```python
from build123d import *

# Parameters (mm, degrees)
SKETCH1_W           = 117.4
SKETCH1_H           = 25.4
BOSS_EXTRUDE1_DEPTH = 1.5875
SKETCH2_W           = 117.4
SKETCH2_H           = 1.5875
BOSS_EXTRUDE2_DEPTH = 23.8125
SKETCH3_R           = 2.54
CUT_EXTRUDE1_DEPTH  = 1.5875
SKETCH4_R           = 2.54
CUT_EXTRUDE2_DEPTH  = 1.5875
FILLET1_R           = 12.7
FILLET2_R           = 3.175


with BuildPart() as part:
    # Sketch1 → Boss-Extrude1 (new body)
    with BuildSketch(Plane.XY):
        with Locations((58.7, 0)):
            Rectangle(SKETCH1_W, SKETCH1_H)
    extrude(amount=BOSS_EXTRUDE1_DEPTH)

    # Sketch2 → Boss-Extrude2 (add)
    with BuildSketch(Plane.XY.offset(1.5875)):
        with Locations((58.7, -11.90625)):
            Rectangle(SKETCH2_W, SKETCH2_H)
    extrude(amount=BOSS_EXTRUDE2_DEPTH)

    # Sketch3 → Cut-Extrude1 (cut)
    with BuildSketch(Plane(origin=(0, -11.1125, 0), x_dir=(1, 0, 0), z_dir=(0, 1, 0))):
        with Locations(Location((12.7, -6.64845, 0), (0, 0, 270))):
            Circle(SKETCH3_R)
        with Locations(Location((104.6990032, -6.64845, 0), (0, 0, 270))):
            Circle(SKETCH3_R)
    extrude(amount=-CUT_EXTRUDE1_DEPTH, mode=Mode.SUBTRACT)

    # Sketch4 → Cut-Extrude2 (cut)
    with BuildSketch(Plane.XY.offset(1.5875)):
        with Locations((18.975, 3.175)):
            Circle(SKETCH4_R)
        with Locations((98.35, 3.175)):
            Circle(SKETCH4_R)
    extrude(amount=-CUT_EXTRUDE2_DEPTH, mode=Mode.SUBTRACT)

    # Fillet1
    fillet1_edges = [part.edges().sort_by_distance(p)[0] for p in [
        (0, -11.90625, 25.4),
        (117.4, -11.90625, 25.4),
    ]]
    fillet(fillet1_edges, radius=FILLET1_R)

    # Fillet2
    fillet2_edges = [part.edges().sort_by_distance(p)[0] for p in [
        (0, 12.7, 0.79375),
        (117.4, 12.7, 0.79375),
    ]]
    fillet(fillet2_edges, radius=FILLET2_R)


solid = part.part
```
Could you check a few things on this model? Use its own coordinates, in mm. A direction names the side the tool comes from. Round coordinates to 2 decimals unless told otherwise and drop trailing zeros. Loops run counter-clockwise (first coordinate to the right, second up) from the corner with the lowest first, then second, coordinate; pieces in that order, holes last. Notation, with made-up numbers: M -33.75,59.25 L -14.75,59.25 A27 ccw -14.75,91.25 Z; hole C 20.25,77.5 d11. An arc over 180 degrees is marked long. Write item = value, one per line.
1. I need wall thicknesses on probe 1 along Z at (x, y) = (36.5, -4); probe 2 along Y at (x, z) = (79, 13); probe 3 along X at (y, z) = (-11.5, 15). Which ranges of each line are inside material? Lowest first, please.
Results below:
probe_1 = 0 to 1.59
probe_2 = -12.7 to -11.11
probe_3 = 0.21 to 117.19
2. Thinking about a two-plate mould opening in Z: for faces 3 (the face through (113.58, -11.9, 21.78)), 4 (the face through (100.696, 2.202, 0.805)), 5 (the face through (15.22, -11.9, 6.32)), which applies, +Z half, -Z half, draft (parallel to the pull), parting line (faces both ways), or undercut?
Results below:
face_3 = +Z half
face_4 = draft
face_5 = undercut
3. Which directions (+Z, -Z, +X, -X, +Y, -Y) give clear straight access to the entire face, cutting with the end or side of a thin tool? Please do faces 1 (the face through (58, -11.112, 13)), 2 (the face through (116.45, 11.79, 0.8)).
Results below:
face_1 = +Z, +X, -X, +Y
face_2 = +Z, -Z, +X, +Y
4. I want a section at D-D, the plane x = 8. Write out the boundary of the cut face in (y, z), and give its area (3 significant figures).
Results below:
outline = M -12.7,0 L 12.7,0 L 12.7,1.59 L -11.11,1.59 L -11.11,24.5 L -12.7,24.5 Z
area = 76.7 mm²
5. I want a section at C-C, the plane z = 17.75. Write out the boundary of the cut face in (x, y).
Results below:
outline = M 1.05,-12.7 L 116.35,-12.7 L 116.35,-11.11 L 1.05,-11.11 Z
6. I want a section at B-B, the plane x = 53.5. Write out the boundary of the cut face in (y, z), and give its area (3 significant figures).
Results below:
outline = M -12.7,0 L 12.7,0 L 12.7,1.59 L -11.11,1.59 L -11.11,25.4 L -12.7,25.4 Z
area = 78.1 mm²
7. Will these pins go through, and if not, where does the flat tip stop? P1, Ø8, axis at x = 12.7, z = 6.65, coming from the +Y side; P2, Ø6.5, axis at x = 18.975, y = 3.175, coming from the +Z side.
Results below:
P1 = -11.11
P2 = 1.59
8. I want a section at A-A, the plane x = 98.35. Write out the boundary of the cut face in (y, z) (1 decimal).
Results below:
outline = M -12.7,0 L 0.6,0 L 0.6,1.6 L -11.1,1.6 L -11.1,25.4 L -12.7,25.4 Z; M 5.7,0 L 12.7,0 L 12.7,1.6 L 5.7,1.6 Z
